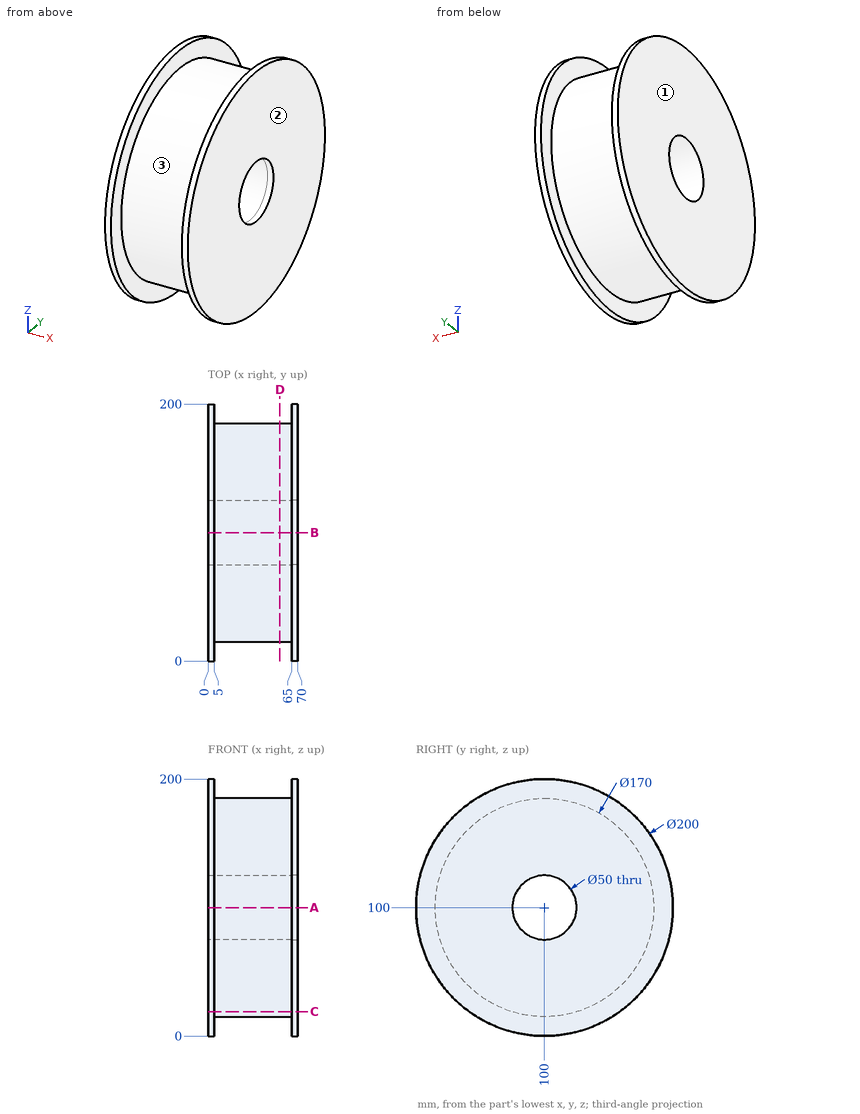
The drawing under review shows one solid part. Ordinate dimensions are in mm from its lowest x, y, z. Coordinates: 2 decimals unless noted, no trailing zeros. Write each loop counter-clockwise with the first axis right and the second up, starting at its lowest first coordinate (ties: lowest second). Pieces come first, ordered by that corner, then holes. Notation, with made-up numbers: M -11.5,12 L 15.5,12 A17 ccw 15.5,39 Z; hole C 1.25,-31 d8. An arc over 180 degrees is marked long. Answer as a JSON object with one key per item and string values.
Item 1: Add section A-A, the plane z = 100. Give the boundary of the cut face in (x, y).
Outcome:
{"outline": "M 0,0 L 5,0 L 5,15 L 65,15 L 65,0 L 70,0 L 70,75 L 0,75 Z; M 0,125 L 70,125 L 70,200 L 65,200 L 65,185 L 5,185 L 5,200 L 0,200 Z"}
Item 2: Insertion check: pin 1 Ø4 at (x, y) = (58, 81) entering from -Z; pin 2 Ø4 at (x, y) = (27, 135.5) entering from +Z; pin 3 Ø4 at (x, z) = (20.5, 95) entering from +Y. Each pin has a flat end and moves straight along its axis. Give the tip position at first contact, or say it passes through.
Outcome:
{"pin 1": "z = 16.72", "pin 2": "z = 178.12", "pin 3": "y = 184.95"}
Item 3: Draft analysis for pull direction X (two halves, no side actions). For the marked faces 1, 2 and 3, state which applies: pulls with the +X half, pulls with the -X half, needs draft (parallel to the pull), parting line crosses it, or undercut.
Outcome:
{"face 1": "pulls with the -X half", "face 2": "pulls with the +X half", "face 3": "undercut"}
Item 4: Add section D-D, the plane x = 56. Give the boundary of the cut face in (y, z).
Outcome:
{"outline": "C 100,100 d170; hole C 100,100 d50"}
Item 5: Add section C-C, the plane z = 19. Give the boundary of the cut face in (x, y).
Outcome:
{"outline": "M 0,41.36 L 5,41.36 L 5,74.23 L 65,74.23 L 65,41.36 L 70,41.36 L 70,158.64 L 65,158.64 L 65,125.77 L 5,125.77 L 5,158.64 L 0,158.64 Z"}
Item 6: Wall thickness on probe 1 along X at (y, z) = (188, 64); probe 2 along Y at (x, z) = (68, 100); probe 3 along Y at (x, z) = (30.5, 100): over which ranges is each line inside the solid? List them lowest first.
Outcome:
{"probe 1": "0 to 5, 65 to 70", "probe 2": "0 to 75, 125 to 200", "probe 3": "15 to 75, 125 to 185"}
